```python
from build123d import *

# Parameters (mm, degrees)
SKETCH1_R           = 9.5
BOSS_EXTRUDE1_DEPTH = 11
SKETCH2_R           = 4
BOSS_EXTRUDE2_DEPTH = 20
FILLET1_R           = 0.6
FILLET2_R           = 0.6


with BuildPart() as part:
    # Sketch1 → Boss-Extrude1 (new body)
    with BuildSketch(Plane.XY):
        Circle(SKETCH1_R)
    extrude(amount=BOSS_EXTRUDE1_DEPTH)

    # Sketch2 → Boss-Extrude2 (add)
    with BuildSketch(Plane(origin=(0, 0, 0), x_dir=(-1, 0, 0), z_dir=(0, 0, -1))):
        Circle(SKETCH2_R)
    extrude(amount=BOSS_EXTRUDE2_DEPTH)

    # Fillet1
    fillet1_edges = [part.edges().sort_by_distance(p)[0] for p in [
        (-9.5, 0, 11),
    ]]
    fillet(fillet1_edges, radius=FILLET1_R)

    # Fillet2
    fillet2_edges = [part.edges().sort_by_distance(p)[0] for p in [
        (-9.5, 0, 0),
    ]]
    fillet(fillet2_edges, radius=FILLET2_R)


solid = part.part
```
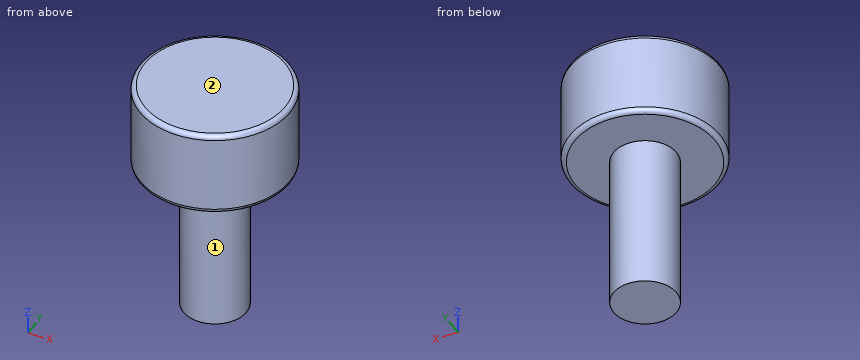
Verification items for the finished model (mm, model axes). Face numbers are marked on the shaded views. A direction names the side the tool comes from. Coordinates: 2 decimals unless noted, no trailing zeros. Write each loop counter-clockwise with the first axis right and the second up, starting at its lowest first coordinate (ties: lowest second). Pieces come first, ordered by that corner, then holes. Notation, with made-up numbers: (87, 89) - (118, 89) arc R12 cw to (118, 97) - close; hole circle Ø10 at (-32, -11.75). An arc over 180 degrees is marked (long way). One line per question, with ' | ' between items. Start each with the question number.
1. Access from +Z, -Z, +X, -X, +Y, -Y to the whole of each face (thin tool, end or side, straight path). Record for the marked faces 1 and 2.
2. Section check C-C (z = -3.5). Enter the section's corners in (x, y), plus the area to 3 significant figures.
3. Section check A-A (x = 0). Enter the section's corners in (y, z).
4. Gauge pin test, flat ends, axial feed: P1, Ø2, axis at y = -7.5, z = 5, coming from the -X side; P2, Ø4, axis at y = 3, z = -9.5, coming from the +X side; P3, Ø2, axis at x = 1.5, z = -4, coming from the +Y side. Record the tip position at first contact, or that the pin passes through.
5. Material ranges on line 1 along Z through (x, y) = (-0.5, 8); line 2 along X through (y, z) = (-0.25, 1.5); line 3 along Y through (x, z) = (-3.5, -1), recorded low to high.
Computed values:
1) face 1: -Z | face 2: +Z, +X, -X, +Y, -Y
2) outline: circle Ø8 at (0, 0) | area: 50.3 mm²
3) outline: (-9.5, 0.6) arc R0.6 ccw to (-8.9, 0) - (-4, 0) - (-4, -20) - (4, -20) - (4, 0) - (8.9, 0) arc R0.6 ccw to (9.5, 0.6) - (9.5, 10.4) arc R0.6 ccw to (8.9, 11) - (-8.9, 11) arc R0.6 ccw to (-9.5, 10.4) - close
4) P1: x = -6.93 | P2: x = 3.87 | P3: y = 3.97
5) line 1: 0 to 11 | line 2: -9.5 to 9.5 | line 3: -1.94 to 1.94
